```python
from build123d import *

# Parameters (mm, degrees)
SKETCH1_R                         = 30
BEARING_DIAMETER_DEPTH            = 10
BEARING_INNER_DIAMETER_DEPTH      = 44.588989435
BEARING_INNER_DIAMETER_DEPTH_BACK = 44.588989435
SKETCH2_R                         = 22.5
CHAMFER1_SIZE                     = 0.25
CHAMFER1_SIZE_2                   = 0.188581226


with BuildPart() as part:
    # Sketch1 → Bearing Diameter (new body)
    with BuildSketch(Plane.XY):
        Circle(SKETCH1_R)
    extrude(amount=BEARING_DIAMETER_DEPTH)

    # Sketch2 → Bearing Inner Diameter (cut, two sides: drawn at the far end of the back side and taken through both)
    with BuildSketch(Plane.XY.offset(10).offset(-BEARING_INNER_DIAMETER_DEPTH_BACK)):
        Circle(SKETCH2_R)
    extrude(amount=BEARING_INNER_DIAMETER_DEPTH + BEARING_INNER_DIAMETER_DEPTH_BACK, mode=Mode.SUBTRACT)

    # Sketch3 → Cut-Revolve2 (revolve, cut)
    with BuildSketch(Plane(origin=(0, 0, 0), x_dir=(1, 0, 0), z_dir=(0, 1, 0))):
        with BuildLine():
            Line((-22.5, 0), (-22.5, -10))
            ThreePointArc((-22.5, -10), (-25.708712153, -5), (-22.5, 0))
        make_face()
    revolve(axis=Axis((0, 0, 0), (0, 0, 1)), mode=Mode.SUBTRACT)

    # Chamfer1
    # the kernel refuses this chamfer: 0.25, 0.188581226 mm, written as the material it takes off along each edge
    with BuildSketch(Plane(origin=(0, 0, 0), x_dir=(-1, 0, 0), z_dir=(0, 1, 0))) as chamfer1_piece_1:
        with BuildLine():
            Line((22.669028641, 0.080971359), (22.5 + CHAMFER1_SIZE, 0))
            Line((22.5 + CHAMFER1_SIZE, 0), (22.5, 0))
            ThreePointArc((22.5, 0), (22.583359545, 0.039047495), (22.669028641, 0.080971359))
        make_face()
    revolve(axis=Axis((0, 0, 0), (0, 0, 1)), mode=Mode.SUBTRACT)
    with BuildSketch(Plane(origin=(0, 0, 10), x_dir=(-1, 0, 0), z_dir=(0, -1, 0))) as chamfer1_piece_2:
        with BuildLine():
            Line((22.5 + CHAMFER1_SIZE_2 * 0.999999998985, 0), (22.730207565, 0.112049419))
            ThreePointArc((22.730207565, 0.112049419), (22.619010369, 0.056270385), (22.5, 0))
            Line((22.5, 0), (22.5 + CHAMFER1_SIZE_2 * 0.999999998985, 0))
        make_face()
    revolve(axis=Axis((0, 0, 10), (0, 0, -1)), mode=Mode.SUBTRACT)
    with BuildSketch(Plane(origin=(0, 0, 0), x_dir=(1, 0, 0), z_dir=(0, -1, 0))) as chamfer1_piece_3:
        Polygon((30, CHAMFER1_SIZE), (30 - CHAMFER1_SIZE, 0), (30, 0), align=None)
    revolve(axis=Axis((0, 0, 0), (0, 0, 1)), mode=Mode.SUBTRACT)
    with BuildSketch(Plane(origin=(0, 0, 10), x_dir=(1, 0, 0), z_dir=(0, -1, 0))) as chamfer1_piece_4:
        Polygon((30, -CHAMFER1_SIZE), (30 - CHAMFER1_SIZE, 0), (30, 0), align=None)
    revolve(axis=Axis((0, 0, 10), (0, 0, 1)), mode=Mode.SUBTRACT)


solid = part.part
```
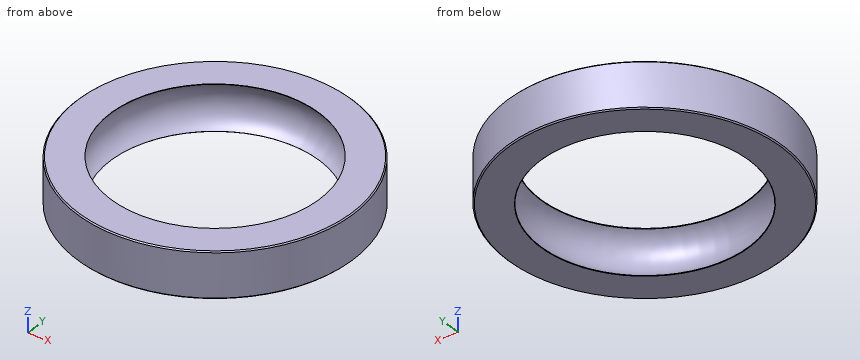
Geometry check sheet. Reference: the model listing, model coordinates, mm. Round coordinates to 2 decimals unless told otherwise and drop trailing zeros. Order: outer loops, then holes, each group sorted by start corner. A loop starts at its lowest first (then second) coordinate and runs counter-clockwise, first axis right, second up. Notation, with made-up numbers: M 37.25,58 L 79.25,58 A12 ccw 79.25,68 Z; hole C 89,3.5 d6. An arc over 180 degrees is marked long. Write item = value, one per line.
Q1. Section check C-C (z = 7). Enter the section's corners in (x, y).
Answer block:
outline = C 0,0 d60; hole C 0,0 d50.66
Q2. Section check D-D (z = 1.5). Enter the section's corners in (x, y).
Answer block:
outline = C 0,0 d60; hole C 0,0 d48.9
Q3. Section check A-A (y = 0). Enter the section's corners in (x, z), plus the area to 3 significant figures.
Answer block:
outline = M -30,0.25 L -29.75,0 L -22.75,0 L -22.67,0.08 A5.5 cw -22.73,9.89 L -22.69,10 L -29.75,10 L -30,9.75 Z; M 22.67,0.08 L 22.75,0 L 29.75,0 L 30,0.25 L 30,9.75 L 29.75,10 L 22.69,10 L 22.73,9.89 A5.5 cw Z
area = 104 mm^2
Q4. Depth check by flat-ended pin: pin 1 Ø6 at (y, z) = (18.5, 5.5) entering from +X; pin 2 Ø3 at (x, z) = (7, 6.5) entering from -Y; pin 3 Ø4 at (x, z) = (-23.5, 7.5) entering from +Y. Enter the tip coordinate at first touch or a pass-through.
Answer block:
pin_1 = 25.69
pin_2 = -29.49
pin_3 = 20.92
Q5. Scan lines: line 1 (X direction, y = -0.5, z = 7.5); line 2 (Z direction, x = 17.5, y = 15); line 3 (X direction, y = 8, z = 6.75). Record each from-to range of solid material in increasing order.
Answer block:
line_1 = -30 to -25.1, 25.1 to 30
line_2 = 0 to 0.29, 9.71 to 10
line_3 = -28.91 to -24.13, 24.13 to 28.91
